Design review of the part shown in the three views and the two pictorial views. Dimensions are in mm from the part's minimum x, y and z. A direction names the side the tool comes from. Round coordinates to 2 decimals unless told otherwise and drop trailing zeros. Write each loop counter-clockwise with the first axis right and the second up, starting at its lowest first coordinate (ties: lowest second). Pieces come first, ordered by that corner, then holes. Notation, with made-up numbers: (18.25, -5.5) - (70.25, -5.5) arc R11 ccw to (70.25, 7.5) - close; hole circle Ø8 at (59, 23.5). An arc over 180 degrees is marked (long way). Use one line per item in the form item = value.
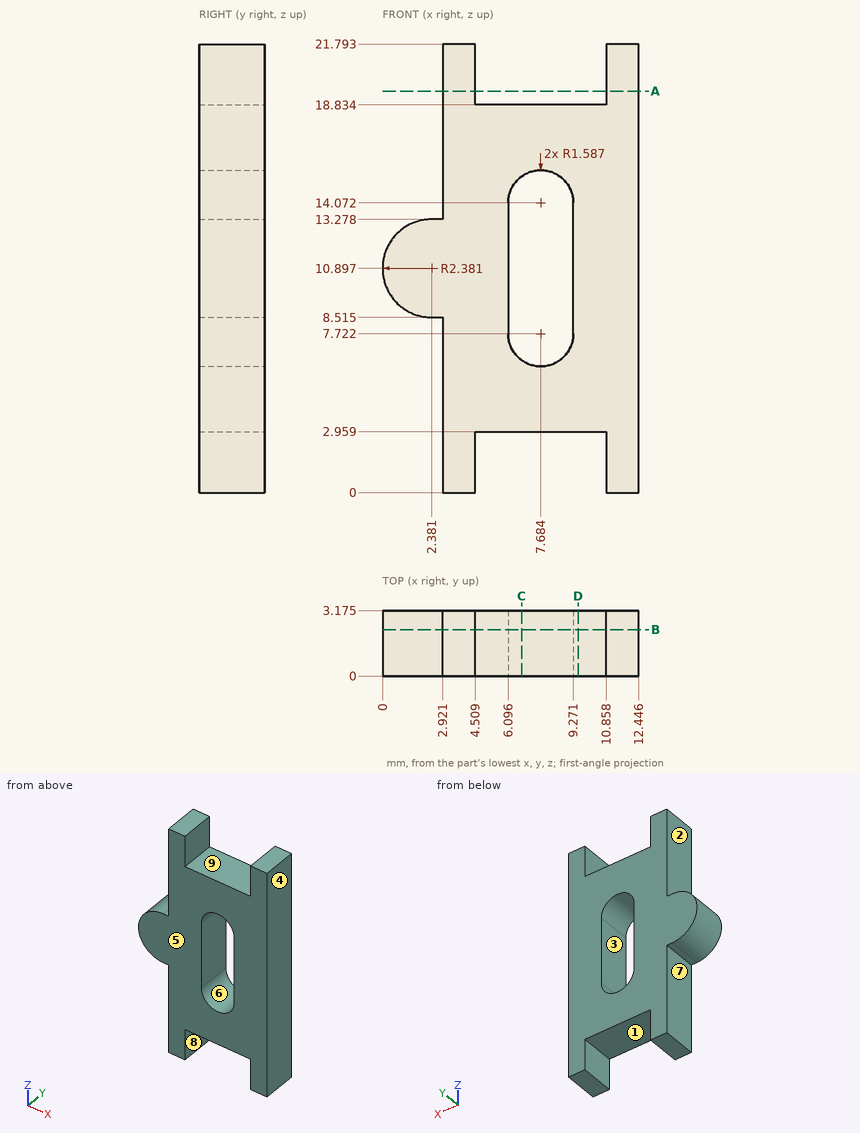
Q1. We need section C-C on x = 6.75. Write out the cut boundary in (y, z) (1 decimal), then the cut area to 3 significant figures.
Calculated:
outline = (0, 3) - (3.2, 3) - (3.2, 6.4) - (0, 6.4) - close; (0, 15.4) - (3.2, 15.4) - (3.2, 18.8) - (0, 18.8) - close
area = 22.1 mm2
Q2. We need section A-A on z = 19.5. Write out the cut boundary in (x, y) (1 decimal).
Calculated:
outline = (2.9, 0) - (4.5, 0) - (4.5, 3.2) - (2.9, 3.2) - close; (10.9, 0) - (12.4, 0) - (12.4, 3.2) - (10.9, 3.2) - close
Q3. To check wall thickness, follow line 1 along X through (y, z) = (0.3, 19.5) (1 decimal); line 2 along X through (y, z) = (2.45, 11) (1 decimal); line 3 along Z through (x, y) = (2.75, 1.85) (1 decimal). State the ranges of each line that lie inside material, in increasing order. Write a range as from..to.
Calculated:
line_1 = 2.9..4.5, 10.9..12.4
line_2 = 0..6.1, 9.3..12.4
line_3 = 8.5..13.3
Q4. We need section D-D on x = 9.5. Write out the cut boundary in (y, z) (1 decimal), then the cut area to 3 significant figures.
Calculated:
outline = (0, 3) - (3.2, 3) - (3.2, 18.8) - (0, 18.8) - close
area = 50.4 mm2
Q5. We need section B-B on y = 2.25. Write out the cut boundary in (x, z) (1 decimal).
Calculated:
outline = (2.4, 8.5) - (2.9, 8.5) - (2.9, 0) - (4.5, 0) - (4.5, 3) - (10.9, 3) - (10.9, 0) - (12.4, 0) - (12.4, 21.8) - (10.9, 21.8) - (10.9, 18.8) - (4.5, 18.8) - (4.5, 21.8) - (2.9, 21.8) - (2.9, 13.3) - (2.4, 13.3) arc R2.4 ccw to start; hole (6.1, 7.7) arc R1.6 ccw to (9.3, 7.7) - (9.3, 14.1) arc R1.6 ccw to (6.1, 14.1) - close
Q6. For P1, Ø1, axis at y = 2, z = 9.5, coming from the -X side (1 decimal); P2, Ø0.9, axis at y = 1, z = 20.5, coming from the -X side; P3, Ø0.6, axis at x = 2.5, y = 1, coming from the +Z side, all flat-tipped, find the tip position at first contact; note any pin that passes through.
Calculated:
P1 = 0.2
P2 = 2.92
P3 = 13.28
Q7. Draft analysis for pull direction X (two halves, no side actions). For the marked faces 1, 2, 3 and 4, state which applies: released by +X, released by -X, zero draft, split by the parting line, or undercut.
Calculated:
face_1 = undercut
face_2 = released by -X
face_3 = undercut
face_4 = released by +X
Q8. Machinability: for the marked faces 5, 6, 7, 8 and 9, which of the approach directions +Z, -Z, +X, -X, +Y, -Y give a long, thin tool a straight path to every point of the face, cutting with its end or side? Answer none if there is none.
Calculated:
face_5 = +Z, -Z, +X, -X, -Y
face_6 = +Y, -Y
face_7 = -Z, -X, +Y, -Y
face_8 = -Z, +Y, -Y
face_9 = +Z, +Y, -Y
